Autodesk Inventor part; units mm, degrees
ref_plane "YZ Plane" through (0, 0, 0) normal (1, 0, 0) x (0, 1, 0)
ref_plane "XZ Plane" through (0, 0, 0) normal (0, 1, 0) x (-1, 0, 0)
ref_plane "XY Plane" through (0, 0, 0) normal (0, 0, 1) x (1, 0, 0)
sketch "Sketch1" plane through (0, 0, 0) normal (0, 0, 1) x (1, 0, 0)
  arc A0 (-24.5511, -4.3997) -> (12.4708, -23.8722) centre (142.4756, 268.2278) ccw
  line L0 (12.4708, -23.8722) -> (31.2882, 11.9043)
  arc A1 (-5.7336, 31.3768) -> (31.2882, 11.9043) centre (142.4756, 268.2278) ccw
  line L1 (-5.7336, 31.3768) -> (-24.5511, -4.3997)
  circle A2 centre (-12.7, 0) radius 4
  circle A3 centre (12.7, 0) radius 2.85
  circle A4 centre (0, 0) radius 2.85
  line L2 (-12.7, 0) -> (12.7, 0) construction
  dimension "d0" = 279.4
  dimension "d1" = 319.7243
  dimension "d2" = 25.4
  dimension "d3" = 40.4234
  dimension "d4" = 40.4234
  dimension "d8" = 31.3768
  dimension "d9" = 4.3997
  dimension "d10" = 18.5882
  dimension "d14" = 5.7
  dimension "d15" = 8
extrude "Extrusion1" add sketch "Sketch1" along normal blind 3.175
properties part number "V5 Shooter Conveyor Spacer 1" material "Aluminum-6061"
Can you work these out from the model? Positions are in its coordinate system, mm. Give positions to 0.01 mm unless a question says otherwise; leave off trailing zeros. Order: outer loops, then holes, each group sorted by start corner. A loop starts at its lowest first (then second) coordinate and runs counter-clockwise, first axis right, second up. Notation, with made-up numbers: M -28.5,40 L 3.5,40 A21 ccw 3.5,64 Z; hole C -30,-37 d10. An arc over 180 degrees is marked long. Write item = value, one per line. Start each with the question number.
Q1. Will this pin go through, and if not, where does the flat tip stop? pin 1 Ø4.5 at (x, y) = (0, 0) entering from -Z.
Q2. Suppose I cut it at D-D (x = 0). Write out the boundary of the cut face in (y, z) (3 decimals), plus the area to 3 significant figures.
Q3. We'd pull the mould along X, two halves only. Please class faces 1 (the cylindrical face through (-6.1, -14.88, 1.57)), 2 (the cylindrical face through (-16.696, -0.176, 1.565)), 3 (the cylindrical face through (15.333, 1.092, 1.565)), 4 (the flat face through (3, 4, 3.175)): pulls with the +X half, pulls with the -X half, needs draft (parallel to the pull), parting line crosses it, or undercut.
Q4. Suppose I cut it at A-A (z = 1.55). Write out the boundary of the cut face in (x, y), plus the area to 3 significant figures.
Q5. Suppose I cut it at C-C (x = -12.7). Write out the boundary of the cut face in (y, z) (3 decimals), plus the area to 3 significant figures.
Q6. I need wall thicknesses on probe 1 along X at (y, z) = (-0.5, 0.9); probe 2 along Y at (x, z) = (-12.7, 1.35); probe 3 along X at (y, z) = (-2, 2.5). Which ranges of each line are inside material? Lowest first, please. Write a range as [from, to].
Q7. Suppose I cut it at B-B (y = 1). Write out the boundary of the cut face in (x, z) (3 decimals), plus the area to 3 significant figures.
Check result:
q1.pin_1 = through
q2.outline = M -17.997,0 L -2.85,0 L -2.85,3.175 L -17.997,3.175 Z; M 2.85,0 L 27.884,0 L 27.884,3.175 L 2.85,3.175 Z
q2.area = 128 mm2
q3.face_1 = pulls with the -X half
q3.face_2 = undercut
q3.face_3 = undercut
q3.face_4 = needs draft
q4.outline = M -24.55,-4.4 A319.72 ccw 12.47,-23.87 L 31.29,11.9 A279.4 cw -5.73,31.38 Z; hole C -12.7,0 d8; hole C 0,0 d5.7; hole C 12.7,0 d5.7
q4.area = 1,590 mm2
q5.outline = M -11.315,0 L -4,0 L -4,3.175 L -11.315,3.175 Z; M 4,0 L 18.132,0 L 18.132,3.175 L 4,3.175 Z
q5.area = 68.1 mm2
q6.probe_1 = [-22.5, -16.67], [-8.73, -2.81], [2.81, 9.89], [15.51, 24.76]
q6.probe_2 = [-11.32, -4], [4, 18.13]
q6.probe_3 = [-23.29, -16.16], [-9.24, -2.03], [2.03, 10.67], [14.73, 23.97]
q7.outline = M -21.711,0 L -16.573,0 L -16.573,3.175 L -21.711,3.175 Z; M -8.827,0 L -2.669,0 L -2.669,3.175 L -8.827,3.175 Z; M 2.669,0 L 10.031,0 L 10.031,3.175 L 2.669,3.175 Z; M 15.369,0 L 25.553,0 L 25.553,3.175 L 15.369,3.175 Z
q7.area = 91.6 mm2
